The listing builds one solid part. Answer for the finished solid, in the listing's coordinates (mm). A direction names the side the tool comes from. Round coordinates to 2 decimals unless told otherwise and drop trailing zeros. Write each loop counter-clockwise with the first axis right and the second up, starting at its lowest first coordinate (ties: lowest second). Pieces come first, ordered by that corner, then holes. Notation, with made-up numbers: (48.25, 22) - (52.25, 22) arc R13 ccw to (52.25, 46) - close; hole circle Ø6 at (7, 11.5). An arc over 180 degrees is marked (long way). Return JSON: item names as keys, results as strings. Group by question number.
(1) Section B-B, the plane y = -52 is taken. Write down the section's boundary in (x, z).
(2) Section A-A, the plane x = -9 is taken. Write down the section's boundary in (y, z), then the cut area to 3 significant figures.
(3) Section C-C, the plane z = -1.75 is taken. Write down the section's boundary in (x, y), then the cut area to 3 significant figures.
(4) Determine the mould class of faces 1 (the flat face through (-9, 1.5, -1)), 2 (the flat face through (0, -1.5, -1)), 3 (the flat face through (14, -34, -1)) for opening direction X: +X half, -X half, draft (parallel to the pull), parting line (faces both ways), or undercut.
(5) Find the intervals of material crossed by line 1 along Y through (x, z) = (0, -0.75); line 2 along Y through (x, z) = (9, -1.6); line 3 along Y through (x, z) = (7.75, -1.25), in increasing order. Write a range as [from, to].
(6) Each of these flat-tipped pins is pushed along its axis until it touches: pin 1 (4 mm diameter, centred on x = -9, y = -56.6, fed in from +Z); pin 2 (2 mm diameter, centred on x = 9, y = -11.4, fed in from -Z). Where does it stop, or does it pass through?
(7) Which of the six approach directions +Z, -Z, +X, -X, +Y, -Y give full straight-line access (tool end or side, diameter ignored) to faces 4 (the cylindrical face through (-0.325, -35.464, -1.479)), 5 (the flat face through (-5, 0, -1)), 6 (the flat face through (0, -66.5, -1))?
(8) Section D-D, the plane x = 0 is taken. Write down the section's boundary in (y, z).
Autodesk Inventor part; units mm, degrees
ref_plane "YZ Plane" through (0, 0, 0) normal (1, 0, 0) x (0, 1, 0)
ref_plane "XZ Plane" through (0, 0, 0) normal (0, 1, 0) x (-1, 0, 0)
ref_plane "XY Plane" through (0, 0, 0) normal (0, 0, 1) x (1, 0, 0)
sketch "Sketch1" plane through (0, 0, 0) normal (0, 0, 1) x (1, 0, 0)
  line L0 (5, 1.5) -> (-5, 1.5)
  line L1 (-5, 1.5) -> (-5, -1.5)
  line L2 (-5, -1.5) -> (5, -1.5)
  line L3 (5, -1.5) -> (5, 1.5)
  line L4 (5, -66.5) -> (-5, -66.5)
  line L5 (-5, -66.5) -> (-5, -69.5)
  line L6 (-5, -69.5) -> (5, -69.5)
  line L7 (5, -69.5) -> (5, -66.5)
  line L8 (14, -1.5) -> (14, 1.5) construction
  line L9 (-14, -1.5) -> (-14, 1.5) construction
  line L10 (-14, -69.5) -> (-14, -66.5) construction
  line L11 (14, -69.5) -> (14, -66.5) construction
  line L12 (14, 1.5) -> (-14, 1.5)
  line L13 (-14, 1.5) -> (-14, -69.5)
  line L14 (-14, -69.5) -> (14, -69.5)
  line L15 (14, -69.5) -> (14, 1.5)
  point P0 (0, 0)
extrude "Extrusion1" add sketch "Sketch1" against normal blind 3 contours L12 L15 L14 L7 L4 L5 L13 L1 L2 L3
sketch "Sketch2" plane through (0, 0, 0) normal (0, 0, 1) x (1, 0, 0)
  line L0 (5, -66.5) -> (5, -69.5) construction
  line L1 (5, -69.5) -> (14, -69.5) construction
  line L2 (14, -69.5) -> (14, 1.5) construction
  line L3 (14, 1.5) -> (5, 1.5) construction
  line L4 (5, 1.5) -> (5, -1.5) construction
  line L5 (5, -1.5) -> (-5, -1.5) construction
  line L6 (-5, -1.5) -> (-5, 1.5) construction
  line L7 (-5, 1.5) -> (-14, 1.5) construction
  line L8 (-14, 1.5) -> (-14, -69.5) construction
  line L9 (-14, -69.5) -> (-5, -69.5) construction
  line L10 (-5, -69.5) -> (-5, -66.5) construction
  line L11 (-5, -66.5) -> (5, -66.5) construction
  line L12 (14, 1.5) -> (-14, -69.5) construction
  line L13 (5, -69.5) -> (14, -69.5) construction
  line L14 (-14, 1.5) -> (14, -69.5) construction
  circle A0 centre (0, -34) radius 1.5
  circle A1 centre (0, -16) radius 1.5
  circle A2 centre (0, -52) radius 1.5
  point P0 (0, 0)
  dimension "d2" = 3
  dimension "d3" = 3
  dimension "d4" = 3
  dimension "d5" = 18
  dimension "d6" = 18
extrude "Extrusion2" cut sketch "Sketch2" against normal blind 3
sketch "Sketch3" plane through (0, 0, -3) normal (0, 0, -1) x (-1, 0, 0)
  circle A0 centre (-9, -56.6) radius 1.8
  circle A1 centre (-9, -11.4) radius 1.8
  circle A2 centre (9, -11.4) radius 1.8
  circle A3 centre (9, -56.6) radius 1.8
  point P0 (0, 0)
extrude "Extrusion3" cut sketch "Sketch3" against normal blind 3
properties part number "Tilt back support with counter balance option"
Working result:
{
 "1": {"outline": "(-14, -3) - (-1.5, -3) - (-1.5, 0) - (-14, 0) - close; (1.5, -3) - (14, -3) - (14, 0) - (1.5, 0) - close"},
 "2": {"outline": "(-69.5, -3) - (-58.4, -3) - (-58.4, 0) - (-69.5, 0) - close; (-54.8, -3) - (-13.2, -3) - (-13.2, 0) - (-54.8, 0) - close; (-9.6, -3) - (1.5, -3) - (1.5, 0) - (-9.6, 0) - close", "area": "191 mm^2"},
 "3": {"outline": "(-14, -69.5) - (-5, -69.5) - (-5, -66.5) - (5, -66.5) - (5, -69.5) - (14, -69.5) - (14, 1.5) - (5, 1.5) - (5, -1.5) - (-5, -1.5) - (-5, 1.5) - (-14, 1.5) - close; hole circle Ø3.6 at (-9, -56.6); hole circle Ø3.6 at (-9, -11.4); hole circle Ø3 at (0, -52); hole circle Ø3 at (0, -34); hole circle Ø3 at (0, -16); hole circle Ø3.6 at (9, -56.6); hole circle Ø3.6 at (9, -11.4)", "area": "1,870 mm^2"},
 "4": {"face 1": "draft", "face 2": "undercut", "face 3": "+X half"},
 "5": {"line 1": "y = [-66.5, -53.5], [-50.5, -35.5], [-32.5, -17.5], [-14.5, -1.5]", "line 2": "y = [-69.5, -58.4], [-54.8, -13.2], [-9.6, 1.5]", "line 3": "y = [-69.5, -57.9], [-55.3, -12.7], [-10.1, 1.5]"},
 "6": {"pin 1": "stops at z = 0", "pin 2": "passes through"},
 "7": {"face 4": "+Z, -Z", "face 5": "+Z, -Z, +Y", "face 6": "+Z, -Z, -Y"},
 "8": {"outline": "(-66.5, -3) - (-53.5, -3) - (-53.5, 0) - (-66.5, 0) - close; (-50.5, -3) - (-35.5, -3) - (-35.5, 0) - (-50.5, 0) - close; (-32.5, -3) - (-17.5, -3) - (-17.5, 0) - (-32.5, 0) - close; (-14.5, -3) - (-1.5, -3) - (-1.5, 0) - (-14.5, 0) - close"}
}
